The listing builds one solid part. Answer for the finished solid, in the listing's coordinates (mm). Face numbers are marked on the shaded views. A direction names the side the tool comes from. Coordinates: 2 decimals unless noted, no trailing zeros. Write each loop counter-clockwise with the first axis right and the second up, starting at its lowest first coordinate (ties: lowest second). Pieces come first, ordered by that corner, then holes. Notation, with made-up numbers: M 78,-8.5 L 120,-8.5 A18 cw 120,19.5 Z; hole C -33.75,83 d6. An arc over 180 degrees is marked long. Write item = value, one per line. Start each with the question number.
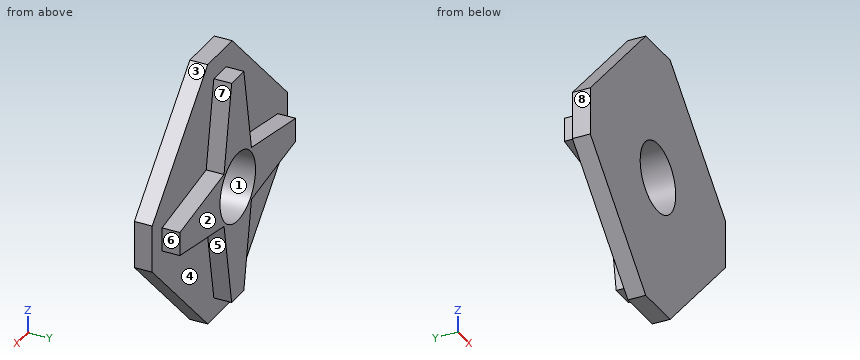
```python
from build123d import *

# Parameters (mm, degrees)
BOSS_EXTRUDE1_DEPTH = 3
BOSS_EXTRUDE2_DEPTH = 3
SKETCH4_R           = 5.829154491
CUT_EXTRUDE3_DEPTH  = 10


with BuildPart() as part:
    # Sketch1 → Boss-Extrude1 (new body)
    with BuildSketch(Plane(origin=(0, 0, 0), x_dir=(1, 0, 0), z_dir=(0, 1, 0))):
        Polygon((-2, 19), (2, 19), (4.5, 4.5), (19, 2), (19, -2), (4.5, -4.5), (2, -19), (-2, -19), (-4.5, -4.5), (-19, -2), (-19, 2), (-4.5, 4.5), align=None)
    extrude(amount=BOSS_EXTRUDE1_DEPTH)

    # Sketch2 → Boss-Extrude2 (add)
    with BuildSketch(Plane(origin=(0, 0, 0), x_dir=(1, 0, 0), z_dir=(0, 1, 0))):
        Polygon((4, 22.483937469), (-4, 22.483937469), (-22.222005883, 4), (-22.222005883, -4), (-4, -22.483937469), (4, -22.483937469), (22.222005883, -4), (22.222005883, 4), align=None)
    extrude(amount=-BOSS_EXTRUDE2_DEPTH)

    # Sketch4 → Cut-Extrude3 (cut, symmetric)
    with BuildSketch(Plane(origin=(0, 0, 0), x_dir=(1, 0, 0), z_dir=(0, 1, 0))):
        with Locations(Location((0, 0, 0), (0, 0, 90))):
            Circle(SKETCH4_R)
    extrude(amount=CUT_EXTRUDE3_DEPTH, both=True, mode=Mode.SUBTRACT)


solid = part.part
```
1. Straight lines are drawn through the part: L1, parallel to X at y = -0.55, z = 0; L2, parallel to X at y = 0.8, z = 0; L3, parallel to Y at x = -4, z = -14. For each, find the intervals that lie inside material, in ascending order. Write a range as [from, to].
2. The part is cut by section A-A, the plane z = 0. Write down the section's boundary in (x, y), and give its area (3 significant figures).
3. The part is cut by section B-B, the plane x = 0. Write down the section's boundary in (y, z), and give its area (3 significant figures).
4. The part is cut by section C-C, the plane y = -0.6. Write down the section's boundary in (x, z), and give its area (3 significant figures).
5. For the marked faces 4, 5, 6, 7 and 8, determine the directions among +Z, -Z, +X, -X, +Y, -Y from which every point of the face is accessible in a straight line to the end or side of a thin tool.
6. Each of these flat-tipped pins is pushed along its axis until it touches: pin 1 (0.9 mm diameter, centred on y = 1.5, z = 0, fed in from -X); pin 2 (1.5 mm diameter, centred on y = 1, z = 0.5, fed in from +X); pin 3 (3 mm diameter, centred on x = 14.5, z = 4.5, fed in from +Y); pin 4 (15 mm diameter, centred on x = 0, z = 0, fed in from +Y). Where does it stop, or does it pass through?
7. The part is cut by section D-D, the plane x = -6.5. Write down the section's boundary in (y, z).
8. For a pull along X with two mould halves and no side action, classify the marked faces 1, 2 and 3 as pulls with the +X half, pulls with the -X half, needs draft (parallel to the pull), parting line crosses it, or undercut.
Solution:
q1.L1 = [-22.22, -5.83], [5.83, 22.22]
q1.L2 = [-19, -5.83], [5.83, 19]
q1.L3 = [-3, 0]
q2.outline = M -22.22,-3 L -5.83,-3 L -5.83,3 L -19,3 L -19,0 L -22.22,0 Z; M 5.83,-3 L 22.22,-3 L 22.22,0 L 19,0 L 19,3 L 5.83,3 Z
q2.area = 177 mm^2
q3.outline = M -3,-22.48 L 0,-22.48 L 0,-19 L 3,-19 L 3,-5.83 L -3,-5.83 Z; M -3,5.83 L 3,5.83 L 3,19 L 0,19 L 0,22.48 L -3,22.48 Z
q3.area = 179 mm^2
q4.outline = M -22.22,-4 L -4,-22.48 L 4,-22.48 L 22.22,-4 L 22.22,4 L 4,22.48 L -4,22.48 L -22.22,4 Z; hole C 0,0 d11.66
q4.area = 1,220 mm^2
q5.face_4 = +Y
q5.face_5 = -Z, +X, +Y
q5.face_6 = +Z, -Z, +X, +Y
q5.face_7 = +Z, +X, +Y
q5.face_8 = +Z, -Z, -X, +Y, -Y
q6.pin_1 = -19
q6.pin_2 = 19
q6.pin_3 = 0
q6.pin_4 = 3
q7.outline = M -3,-19.95 L 0,-19.95 L 0,-4.16 L 3,-4.16 L 3,4.16 L 0,4.16 L 0,19.95 L -3,19.95 Z
q8.face_1 = undercut
q8.face_2 = needs draft
q8.face_3 = pulls with the +X half
